Can you work these out from the model? Positions are in its coordinate system, mm. A direction names the side the tool comes from. Give positions to 0.01 mm unless a question says otherwise; leave off trailing zeros. Order: outer loops, then holes, each group sorted by start corner. A loop starts at its lowest first (then second) coordinate and runs counter-clockwise, first axis right, second up. Notation, with made-up numbers: (62.25, 70.25) - (111.25, 70.25) arc R29 ccw to (111.25, 92.25) - close; hole circle Ø8 at (-35, 79). An arc over 180 degrees is marked (long way). One line per question, with ' | ' between items.
```python
from build123d import *

# Parameters (mm, degrees)
F1_DEPTH = 500
F2_SIZE  = 0.5


with BuildPart() as f1:
    # F0 (on Top) → F1 (new body)
    with BuildSketch(Plane.XY):
        with BuildLine():
            Line((-30, 50), (-50, 50))
            Line((-50, 50), (-50, 30))
            Line((-50, 30), (-44, 30))
            Line((-44, 30), (-44, 35))
            Line((-44, 35), (-37, 35))
            Line((-37, 35), (-37, 25.5))
            Line((-37, 25.5), (-30.97913, 25.5))
            ThreePointArc((-30.97913, 25.5), (-29.242641, 29.242641), (-25.5, 30.97913))
            ThreePointArc((-25.5, 30.97913), (-20.408156, 28.861991), (-19.195037, 23.482633))
            Line((-19.195037, 23.482633), (-12.5, 30.17767))
            Line((-12.5, 30.17767), (12.5, 30.17767))
            Line((12.5, 30.17767), (19.195037, 23.482633))
            ThreePointArc((19.195037, 23.482633), (29.242641, 29.242641), (23.482633, 19.195037))
            Line((23.482633, 19.195037), (30.17767, 12.5))
            Line((30.17767, 12.5), (30.17767, -12.5))
            Line((30.17767, -12.5), (23.482633, -19.195037))
            ThreePointArc((23.482633, -19.195037), (29.242641, -29.242641), (19.195037, -23.482633))
            Line((19.195037, -23.482633), (12.5, -30.17767))
            Line((12.5, -30.17767), (-12.5, -30.17767))
            Line((-12.5, -30.17767), (-19.195037, -23.482633))
            ThreePointArc((-19.195037, -23.482633), (-29.242641, -29.242641), (-23.482633, -19.195037))
            Line((-23.482633, -19.195037), (-30.17767, -12.5))
            Line((-30.17767, -12.5), (-30.17767, 12.5))
            Line((-30.17767, 12.5), (-23.482633, 19.195037))
            ThreePointArc((-23.482633, 19.195037), (-28.465904, 20.102295), (-30.97913, 24.5))
            Line((-30.97913, 24.5), (-37, 24.5))
            Line((-37, 24.5), (-37, 15))
            Line((-37, 15), (-44, 15))
            Line((-44, 15), (-44, 20))
            Line((-44, 20), (-50, 20))
            Line((-50, 20), (-50, -20))
            Line((-50, -20), (-44, -20))
            Line((-44, -20), (-44, -15))
            Line((-44, -15), (-37, -15))
            Line((-37, -15), (-37, -35))
            Line((-37, -35), (-44, -35))
            Line((-44, -35), (-44, -30))
            Line((-44, -30), (-50, -30))
            Line((-50, -30), (-50, -50))
            Line((-50, -50), (-30, -50))
            Line((-30, -50), (-30, -44))
            Line((-30, -44), (-35, -44))
            Line((-35, -44), (-35, -37))
            Line((-35, -37), (-15, -37))
            Line((-15, -37), (-15, -44))
            Line((-15, -44), (-20, -44))
            Line((-20, -44), (-20, -50))
            Line((-20, -50), (20, -50))
            Line((20, -50), (20, -44))
            Line((20, -44), (15, -44))
            Line((15, -44), (15, -37))
            Line((15, -37), (35, -37))
            Line((35, -37), (35, -44))
            Line((35, -44), (30, -44))
            Line((30, -44), (30, -50))
            Line((30, -50), (50, -50))
            Line((50, -50), (50, -30))
            Line((50, -30), (44, -30))
            Line((44, -30), (44, -35))
            Line((44, -35), (37, -35))
            Line((37, -35), (37, -15))
            Line((37, -15), (44, -15))
            Line((44, -15), (44, -20))
            Line((44, -20), (50, -20))
            Line((50, -20), (50, 20))
            Line((50, 20), (44, 20))
            Line((44, 20), (44, 15))
            Line((44, 15), (37, 15))
            Line((37, 15), (37, 35))
            Line((37, 35), (44, 35))
            Line((44, 35), (44, 30))
            Line((44, 30), (50, 30))
            Line((50, 30), (50, 50))
            Line((50, 50), (30, 50))
            Line((30, 50), (30, 44))
            Line((30, 44), (35, 44))
            Line((35, 44), (35, 37))
            Line((35, 37), (15, 37))
            Line((15, 37), (15, 44))
            Line((15, 44), (20, 44))
            Line((20, 44), (20, 50))
            Line((20, 50), (-20, 50))
            Line((-20, 50), (-20, 44))
            Line((-20, 44), (-15, 44))
            Line((-15, 44), (-15, 37))
            Line((-15, 37), (-25.5, 37))
            Line((-25.5, 37), (-35, 37))
            Line((-35, 37), (-35, 44))
            Line((-35, 44), (-30, 44))
            Line((-30, 44), (-30, 50))
        make_face()
    extrude(amount=F1_DEPTH)

    # F2
    f2_edges = [f1.edges().sort_by_distance(p)[0] for p in [
        (-23.987564, 30.913964, 500),
        (-28.465904, 20.102295, 500),
        (-29.242641, -29.242641, 500),
        (29.242641, -29.242641, 500),
        (29.242641, 29.242641, 500),
        (29.242641, 29.242641, 0),
        (29.242641, -29.242641, 0),
        (-29.242641, -29.242641, 0),
        (-28.465904, 20.102295, 0),
        (-23.987564, 30.913964, 0),
    ]]
    chamfer(f2_edges, length=F2_SIZE)


solid = f1.part
```
(1) If we mould it in two halves opening along Y, with no side actions, what happens to faces 3 (the face through (0, 50, 246)), 4 (the face through (-30.178, 0, 246)), 5 (the face through (-50, 0, 246))? For each: released by +Y, released by -Y, zero draft, split by the parting line, or undercut.
Answer below:
face 3: released by +Y | face 4: undercut | face 5: zero draft
(2) If I drill on line 1 (Y direction, x = 34, z = 33); line 2 (Y direction, x = 44.5, z = 198); line 3 (Y direction, x = -33.5, z = 267.5), over which ranges is the centre line in solid material (lowest first)?
Answer below:
line 1: -50 to -44, -37 to 37, 44 to 50 | line 2: -50 to -30, -20 to 20, 30 to 50 | line 3: -50 to -44, -37 to 24.5, 25.5 to 37, 44 to 50
(3) Imagine slicing it at A-A (y = -4.5). List the corners of the cut face in (x, z) for me.
Answer below:
outline: (-50, 0) - (-30.18, 0) - (-30.18, 500) - (-50, 500) - close; (30.18, 0) - (50, 0) - (50, 500) - (30.18, 500) - close
(4) On a 3-axis mill with a long thin cutter (end or side, diameter ignored), from which of +Z, -Z, +X, -X, +Y, -Y can I reach the whole of each face in a straight line? I mean faces 1 (the face through (50, 40, 246)), 2 (the face through (-25, -37, 246)). Say none if no direction works.
Answer below:
face 1: +Z, -Z, +X, +Y, -Y | face 2: +Z, -Z
